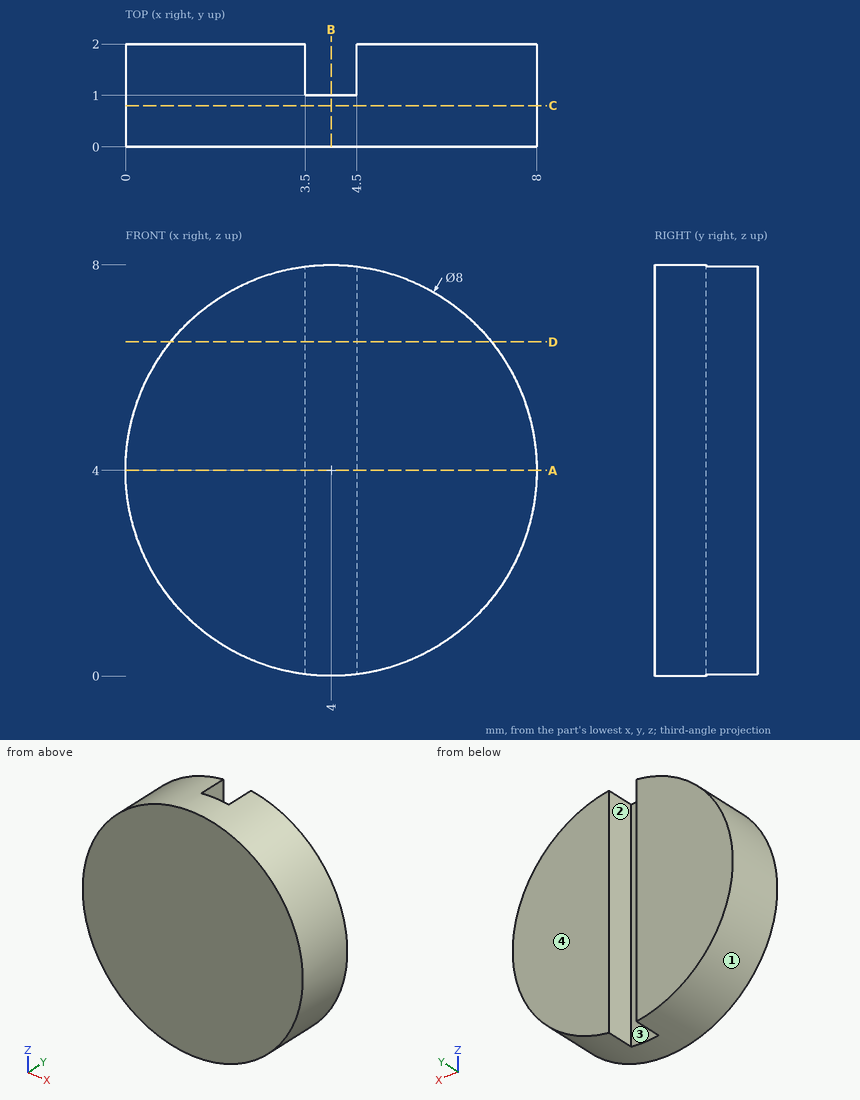
Source: three-view drawing plus pictorial views. Frame: mm from the lowest corner of the part. Coordinates: 2 decimals unless noted, no trailing zeros. Order: outer loops, then holes, each group sorted by start corner. A loop starts at its lowest first (then second) coordinate and runs counter-clockwise, first axis right, second up. Notation, with made-up numbers: M 17,88.5 L 54,88.5 A30 cw 54,115.5 Z; hole C -8.5,-8 d11. An arc over 180 degrees is marked long. One line per question, with ' | ' between items.
Item 1: Section A-A (z = 4). Output: boundary loops of the cut face in (x, y).
Geometry results:
outline: M 0,0 L 8,0 L 8,2 L 4.5,2 L 4.5,1 L 3.5,1 L 3.5,2 L 0,2 Z
Item 2: Ray query, line 1 along X through (y, z) = (1.1, 4); line 2 along X through (y, z) = (1.65, 6.5); line 3 along Y through (x, z) = (4, 2.5). Return the intervals inside material, ascending.
Geometry results:
line 1: x = 0 to 3.5, 4.5 to 8 | line 2: x = 0.88 to 3.5, 4.5 to 7.12 | line 3: y = 0 to 1
Item 3: Pin query (flat end, axial travel): pin 1 (1.1 mm diameter, centred on y = 1.5, z = 3, fed in from +X). Return the tip coordinate at first contact, or that it passes through.
Geometry results:
pin 1: stops at x = 7.97
Item 4: Section C-C (y = 0.8). Output: boundary loops of the cut face in (x, z).
Geometry results:
outline: C 4,4 d8
Item 5: Section D-D (z = 6.5). Output: boundary loops of the cut face in (x, y), then the cut area to 3 significant figures.
Geometry results:
outline: M 0.88,0 L 7.12,0 L 7.12,2 L 4.5,2 L 4.5,1 L 3.5,1 L 3.5,2 L 0.88,2 Z | area: 11.5 mm^2
Item 6: Section B-B (x = 4). Output: boundary loops of the cut face in (y, z).
Geometry results:
outline: M 0,0 L 1,0 L 1,8 L 0,8 Z
Item 7: Draft query along X for the marked faces 1, 2, 3 and 4. Return one class per face: released by +X, released by -X, zero draft, split by the parting line, or undercut.
Geometry results:
face 1: split by the parting line | face 2: undercut | face 3: undercut | face 4: zero draft
